Source: CAD feature listing. Evaluate the final solid. Frame: model axes, mm. Face numbers are marked on the shaded views. Give positions to 0.01 mm unless a question says otherwise; leave off trailing zeros. Write each loop counter-clockwise with the first axis right and the second up, starting at its lowest first coordinate (ties: lowest second). Pieces come first, ordered by that corner, then holes. Notation, with made-up numbers: (-38, 12) -> (-4, 12) arc R21 ccw to (-4, 17) -> close; hole circle Ø6 at (81, -37). An arc over 180 degrees is marked (long way). Use one line per item in the form item = value. Start each with the question number.
(1) Draft query along X for the marked faces 1, 2 and 3. Return one class per face: pulls with the +X half, pulls with the -X half, needs draft (parallel to the pull), parting line crosses it, or undercut.
(2) Cut plane D-D, the plane z = 10.5. Output: boundary loops of the cut face in (x, y).
(3) Material intervals for line 1 along Z through (x, y) = (0, 18.3); line 2 along X through (y, z) = (11.25, -1.25); line 3 along X through (y, z) = (16.75, -2.75), sorted ascending. Write a range as from..to.
(4) Cut plane B-B, the plane z = 1. Output: boundary loops of the cut face in (x, y).
(5) First-contact query: P1, Ø1, axis at y = 4, z = -5.5, coming from the -X side; P2, Ø1, axis at y = 4.5, z = 1, coming from the -X side; P3, Ø5.5, axis at x = 0, z = 0, coming from the -Y side; P4, Ø5, axis at y = 7.5, z = -8.5, coming from the +X side. Flat tips, straight axial feed; report the tip coordinate or a pass-through.
(6) Cut plane A-A, the plane x = 0. Output: boundary loops of the cut face in (y, z) (1 decimal), and give its area (3 significant figures).
(7) Cut plane C-C, the plane y = 14.5. Output: boundary loops of the cut face in (x, z), and give its area (3 significant figures).
Autodesk Inventor part; units mm, degrees
ref_plane "YZ Plane" through (0, 0, 0) normal (1, 0, 0) x (0, 1, 0)
ref_plane "XZ Plane" through (0, 0, 0) normal (0, 1, 0) x (-1, 0, 0)
ref_plane "XY Plane" through (0, 0, 0) normal (0, 0, 1) x (1, 0, 0)
sketch "Sketch1" plane through (0, 0, 0) normal (0, 1, 0) x (-1, 0, 0)
  circle A0 centre (0, 0) radius 12.7
  circle A1 centre (0, 0) radius 3.302
  dimension "d0" = 25.4
  dimension "d1" = 6.604
extrude "Extrusion1" add sketch "Sketch1" along normal blind 19.5732
sketch "Sketch2" plane through (0, 19.5732, 0) normal (0, 1, 0) x (1, 0, 0)
  line L0 (0, 0) -> (0, -5.004)
  line L1 (0, -5.004) -> (0, 0)
  line L2 (0, 0) -> (0, 5.004)
  circle A0 centre (0, -5.004) radius 1.0125
  circle A1 centre (0, 5.004) radius 1.0125
  dimension "d4" = 5.004
  dimension "d5" = 5.004
  dimension "d6" = 2.025
  dimension "d7" = 2.025
extrude "Extrusion2" cut sketch "Sketch2" against normal blind 4.445
sketch "Sketch3" plane through (0, 0, 0) normal (0, -1, 0) x (1, 0, 0)
  line L0 (0, 0) -> (0, 5.004)
  circle A0 centre (0, 5.004) radius 1.0125
  line L1 (0, 0) -> (0, -5.004)
  circle A1 centre (0, -5.004) radius 1.0125
  dimension "d10" = 5.004
  dimension "d15" = 2.025
  dimension "d16" = 5.004
  dimension "d17" = 2.025
extrude "Extrusion3" cut sketch "Sketch3" against normal blind 4.445
properties part number "PolarisPost_HeightAdjustment_0p77in_ForK1S4Mirrors_Machined"
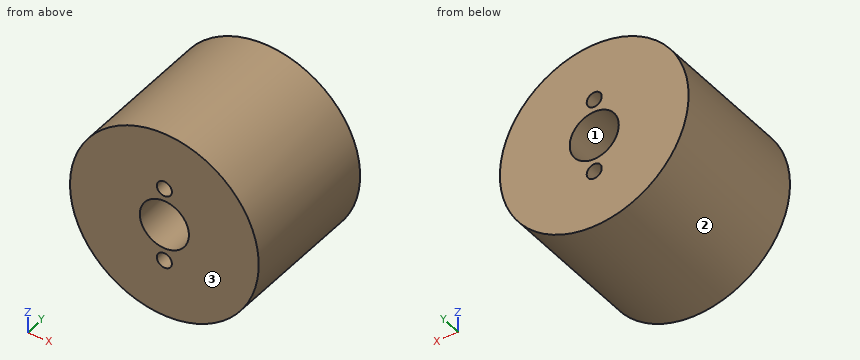
Geometry says:
q1.face_1 = undercut
q1.face_2 = parting line crosses it
q1.face_3 = needs draft
q2.outline = (-7.14, 0) -> (7.14, 0) -> (7.14, 19.57) -> (-7.14, 19.57) -> close
q3.line_1 = -12.7..-6.02, -3.99..-3.3, 3.3..3.99, 6.02..12.7
q3.line_2 = -12.64..-3.06, 3.06..12.64
q3.line_3 = -12.4..-1.83, 1.83..12.4
q4.outline = (-12.66, 0) -> (-3.15, 0) -> (-3.15, 19.57) -> (-12.66, 19.57) -> close; (3.15, 0) -> (12.66, 0) -> (12.66, 19.57) -> (3.15, 19.57) -> close
q5.P1 = -11.67
q5.P2 = -12.69
q5.P3 = through
q5.P4 = 11.19
q6.outline = (0, -12.7) -> (19.6, -12.7) -> (19.6, -6) -> (15.1, -6) -> (15.1, -4) -> (19.6, -4) -> (19.6, -3.3) -> (0, -3.3) -> (0, -4) -> (4.4, -4) -> (4.4, -6) -> (0, -6) -> close; (0, 3.3) -> (19.6, 3.3) -> (19.6, 4) -> (15.1, 4) -> (15.1, 6) -> (19.6, 6) -> (19.6, 12.7) -> (0, 12.7) -> (0, 6) -> (4.4, 6) -> (4.4, 4) -> (0, 4) -> close
q6.area = 332 mm^2
q7.outline = circle Ø25.4 at (0, 0); hole circle Ø6.6 at (0, 0)
q7.area = 472 mm^2
